Design review of the part built by this model. Coordinates are the model's own, in mm. A direction names the side the tool comes from. Coordinates: 2 decimals unless noted, no trailing zeros. Loops run counter-clockwise (first coordinate to the right, second up) from the corner with the lowest first, then second, coordinate; pieces in that order, holes last.
Q1. Machinability: for faces 1 (the face through (-156, 0, 0)), 2 (the face through (164.374, 3.648, -135.181)), which of the approach directions +Z, -Z, +X, -X, +Y, -Y give a long, thin tool a straight path to every point of the face, cutting with its end or side? Answer none if there is none.
Q2. Add section B-B on x = -24.5. Give the boundary of the cut face in (y, z) (3 decimals), and give its area (3 significant figures).
Q3. For P1, Ø10, axis at y = 0, z = -203.2, coming from the -X side, flat-tipped, find the tip position at first contact; note if it passes through.
Q4. Wall thickness on probe 1 along Y at (x, z) = (-156.25, -203.2) (3 decimals); probe 2 along Z at (x, y) = (-157.75, 0) (3 decimals); probe 3 along Y at (x, z) = (-158.75, -203.2) (3 decimals): over which ranges is each line inside the solid? List them lowest first.
Q5. Draft analysis for pull direction X (two halves, no side actions). For faces 3 (the face through (156, 0, 0)), 4 (the face through (-164.374, 3.648, -135.181)), state which applies: released by +X, released by -X, zero draft, split by the parting line, or undercut.
Q6. Add section A-A on z = -47.5. Give the boundary of the cut face in (x, y) (3 decimals).
```python
from build123d import *

# Parameters (mm, degrees)
SWEEP1_PROFILE_R   = 9.525
SWEEP2_PROFILE_R   = 9.525
SKETCH37_R         = 3.175
CUT_EXTRUDE1_DEPTH = 405.640507596


with BuildPart() as part:
    # Sweep1: sweep along a path in Sketch2
    with BuildLine(Plane(origin=(0, -28.669314133, -327.691760022), x_dir=(-1, 0, 0), z_dir=(0, 0.08715574274765835, 0.9961946980917455))) as sweep1_path:
        Line((0, -139.683627769), (28.771853902, -139.683627769))
        ThreePointArc((28.771853902, -139.683627769), (56.13800648, -130.260705766), (71.901498935, -105.987056028))
        Line((71.901498935, -105.987056028), (91.151672667, -28.778826255))
    # Sweep1 profile (on start of the path) → Sweep1 (sweep)
    with BuildSketch(Plane(origin=(0, 110.482775261, -339.86599035), x_dir=(0, 0, -1), z_dir=(-1, 0, 0))):
        Circle(SWEEP1_PROFILE_R)
    sweep1 = sweep(path=sweep1_path.line)

    # Sweep2: sweep along a path in Sketch1
    with BuildLine(Plane(origin=(0, 0, 0), x_dir=(1, 0, 0), z_dir=(0, 1, 0))) as sweep2_path:
        Line((0, 330.2), (-99.575, 330.2))
        ThreePointArc((-99.575, 330.2), (-139.172979746, 313.797979746), (-155.575, 274.2))
        Line((-155.575, 274.2), (-155.575, 0))
    # Sweep2 profile (on start of the path) → Sweep2 (sweep)
    with BuildSketch(Plane(origin=(0, 0, -330.2), x_dir=(0, 0, -1), z_dir=(-1, 0, 0))):
        Circle(SWEEP2_PROFILE_R)
    sweep2 = sweep(path=sweep2_path.line)

    # Sketch37 → Cut-Extrude1 (cut, through all)
    with BuildSketch(Plane(origin=(0, 0, 0), x_dir=(0, 0, -1), z_dir=(1, 0, 0))):
        with Locations((203.2, 0)):
            Circle(SKETCH37_R)
    cut_extrude1 = extrude(amount=-CUT_EXTRUDE1_DEPTH, mode=Mode.SUBTRACT)

    # Mirror1: Sweep1, Sweep2, Cut-Extrude1 across plane
    add(sweep1.mirror(Plane(origin=(0, 0, 0), x_dir=(0, 0, 1), z_dir=(1, 0, 0))))
    add(sweep2.mirror(Plane(origin=(0, 0, 0), x_dir=(0, 0, 1), z_dir=(1, 0, 0))))
    add(cut_extrude1.mirror(Plane(origin=(0, 0, 0), x_dir=(0, 0, 1), z_dir=(1, 0, 0))), mode=Mode.SUBTRACT)


solid = part.part
```
Entries:
1. face 1: +Z, +X, -X, +Y, -Y
1. face 2: +Z
2. outline: circle Ø19.05 at (0, -330.2); circle Ø19.05 at (110.483, -339.866)
2. area: 570 mm2
3. P1: stops at x = -165.1
4. probe 1: y = -9.501 to -3.175, 3.175 to 9.501
4. probe 2: z = -304.353 to -206.375, -200.025 to 0
4. probe 3: y = -8.98 to -3.175, 3.175 to 8.98
5. face 3: zero draft
5. face 4: undercut
6. outline: circle Ø19.05 at (-155.575, 0); circle Ø19.05 at (155.575, 0)
